```python
from build123d import *

# Parameters (mm, degrees)
SKETCH_1_W          = 175
SKETCH_1_H          = 63
EXTRUDE_1_DEPTH     = 5
CUT_EXTRUDE_1_DEPTH = 5
CHAMFER_1_SIZE      = 15
CHAMFER_2_SIZE      = 5
EXTRUDE_START       = -7
EXTRUDE_2_DEPTH     = 25
EXTRUDE_START_2     = -12
SKETCH_5_W          = 68
SKETCH_5_H          = 5
SKETCH_5_W_2        = 70
EXTRUDE_4_DEPTH     = 2
FILLET_1_R          = 3
FILLET_2_R          = 3
FILLET_3_R          = 1


with BuildPart() as part:
    # 草图1 → 凸台-拉伸1 (new body)
    with BuildSketch(Plane.XY):
        with Locations((0, 24.5)):
            Rectangle(SKETCH_1_W, SKETCH_1_H)
    extrude(amount=EXTRUDE_1_DEPTH)

    # 草图2 → 切除-拉伸1 (cut)
    with BuildSketch(Plane.XY.offset(5)):
        Polygon((-75, 56), (-4, 56), (-4, 43.171572875), (-10.171572875, 37), (-68.828427125, 37), (-75, 43.171572875), align=None)
    extrude(amount=-CUT_EXTRUDE_1_DEPTH, mode=Mode.SUBTRACT)

    # 倒角1
    chamfer_1_edges = [part.edges().sort_by_distance(p)[0] for p in [
        (87.5, -7, 2.5),
        (-87.5, -7, 2.5),
    ]]
    chamfer(chamfer_1_edges, length=CHAMFER_1_SIZE)

    # 倒角2
    chamfer_2_edges = [part.edges().sort_by_distance(p)[0] for p in [
        (-87.5, 56, 2.5),
        (87.5, 56, 2.5),
    ]]
    chamfer(chamfer_2_edges, length=CHAMFER_2_SIZE)

    # 草图4 → 凸台-拉伸2 (add)
    with BuildSketch(Plane.XZ.offset(7).offset(EXTRUDE_START)):
        Polygon((-23.5, -3), (-53.5, -3), (-51.767949192, 0), (-25.232050808, 0), align=None)
        Polygon((23.5, -3), (25.232050808, 0), (51.767949192, 0), (53.5, -3), align=None)
    extrude(amount=-EXTRUDE_2_DEPTH)

    # 草图5 → 凸台-拉伸4 (add)
    with BuildSketch(Plane(origin=(0, 37, 0), x_dir=(1, 0, 0), z_dir=(0, 1, 0)).offset(EXTRUDE_START_2)):
        with Locations((-39.5, 2.5)):
            Rectangle(SKETCH_5_W, SKETCH_5_H)
        with Locations((38.5, 2.5)):
            Rectangle(SKETCH_5_W_2, SKETCH_5_H)
    extrude(amount=-EXTRUDE_4_DEPTH)

    # 圆角1
    fillet_1_edges = [part.edges().sort_by_distance(p)[0] for p in [
        (-4, 43.171572875, 2.5),
        (-10.171572875, 37, 2.5),
        (-68.828427125, 37, 2.5),
        (-75, 43.171572875, 2.5),
        (-75, 56, 2.5),
        (-4, 56, 2.5),
        (72.5, -7, 2.5),
        (-72.5, -7, 2.5),
        (-87.5, 8, 2.5),
        (87.5, 8, 2.5),
        (82.5, 56, 2.5),
        (87.5, 51, 2.5),
        (-82.5, 56, 2.5),
    ]]
    fillet(fillet_1_edges, radius=FILLET_1_R)

    # 圆角2
    fillet_2_edges = [part.edges().sort_by_distance(p)[0] for p in [
        (-87.5, 51, 2.5),
    ]]
    fillet(fillet_2_edges, radius=FILLET_2_R)

    # 圆角3
    fillet_3_edges = [part.edges().sort_by_distance(p)[0] for p in [
        (40.128679656, 56, 5),
        (40.128679656, 56, 0),
        (87.5, 29.5, 5),
        (85, 53.5, 5),
        (-4, 48.707106781, 5),
        (-7.085786438, 40.085786438, 5),
        (-39.5, 37, 5),
        (-71.914213562, 40.085786438, 5),
        (-75, 48.707106781, 5),
        (-79.628679656, 56, 5),
        (-85, 53.5, 5),
        (-80, 0.5, 5),
        (0, -7, 5),
        (80, 0.5, 5),
        (-82.40540961, 55.771638598, 5),
        (-87.271638598, 8.09459039, 5),
        (-72.40540961, -6.771638598, 5),
        (82.40540961, 55.771638598, 5),
        (87.271638598, 50.90540961, 5),
        (87.271638598, 8.09459039, 5),
        (72.40540961, -6.771638598, 5),
        (-75.878679656, 55.121320344, 5),
        (-3.121320344, 55.121320344, 5),
        (-4, 48.707106781, 0),
        (85, 53.5, 0),
        (87.5, 29.5, 0),
        (80, 0.5, 0),
        (0, -7, 0),
        (-80, 0.5, 0),
        (-79.628679656, 56, 0),
        (-75, 48.707106781, 0),
        (-71.914213562, 40.085786438, 0),
        (-39.5, 37, 0),
        (-7.085786438, 40.085786438, 0),
        (-82.40540961, 55.771638598, 0),
        (-87.271638598, 8.09459039, 0),
        (-72.40540961, -6.771638598, 0),
        (82.40540961, 55.771638598, 0),
        (87.271638598, 50.90540961, 0),
        (87.271638598, 8.09459039, 0),
        (72.40540961, -6.771638598, 0),
        (-75.878679656, 55.121320344, 0),
        (-3.121320344, 55.121320344, 0),
        (-4.228361402, 43.266163265, 5),
        (-4.228361402, 43.266163265, 0),
        (-10.266163265, 37.228361402, 5),
        (-10.266163265, 37.228361402, 0),
        (-68.733836735, 37.228361402, 5),
        (-68.733836735, 37.228361402, 0),
        (-74.771638598, 43.266163265, 5),
        (-74.771638598, 43.266163265, 0),
        (-87.5, 29.5, 0),
        (-87.5, 29.5, 5),
        (-85, 53.5, 0),
        (-87.271638598, 50.90540961, 0),
        (-87.271638598, 50.90540961, 5),
    ]]
    fillet(fillet_3_edges, radius=FILLET_3_R)


solid = part.part
```
Input: part model. Units: mm. Frame: model coordinates. A direction names the side the tool comes from. Give positions to 0.01 mm unless a question says otherwise; leave off trailing zeros. Order: outer loops, then holes, each group sorted by start corner. A loop starts at its lowest first (then second) coordinate and runs counter-clockwise, first axis right, second up.
1. Line query: probe 1 along Y at (x, z) = (-21.5, -4.5); probe 2 along Z at (x, y) = (-49.5, 10.5); probe 3 along Z at (x, y) = (-49.5, 29). Output: solid intervals per line, ascending.
Computed:
probe 1: y = 23 to 25
probe 2: z = -3 to 5
probe 3: z = 0 to 5
2. Cut plane A-A (y = 19). Return loops of the section in (x, z), and give its area (3 significant figures).
Computed:
outline: (-87.5, 1) arc R1 ccw to (-86.5, 0) - (-51.77, 0) - (-53.5, -3) - (-23.5, -3) - (-25.23, 0) - (25.23, 0) - (23.5, -3) - (53.5, -3) - (51.77, 0) - (86.5, 0) arc R1 ccw to (87.5, 1) - (87.5, 4) arc R1 ccw to (86.5, 5) - (-86.5, 5) arc R1 ccw to (-87.5, 4) - close
area: 1,040 mm2
3. Cut plane C-C (x = 65). Return loops of the section in (y, z).
Computed:
outline: (-7, 1) arc R1 ccw to (-6, 0) - (23, 0) - (23, -5) - (25, -5) - (25, 0) - (55, 0) arc R1 ccw to (56, 1) - (56, 4) arc R1 ccw to (55, 5) - (-6, 5) arc R1 ccw to (-7, 4) - close
4. Cut plane B-B (z = -1.5). Return loops of the section in (x, y).
Computed:
outline: (-73.5, 23) - (-52.63, 23) - (-52.63, 0) - (-24.37, 0) - (-24.37, 23) - (-5.5, 23) - (-5.5, 25) - (-73.5, 25) - close; (3.5, 23) - (24.37, 23) - (24.37, 0) - (52.63, 0) - (52.63, 23) - (73.5, 23) - (73.5, 25) - (3.5, 25) - close
5. Cut plane D-D (y = 30). Return loops of the section in (x, z).
Computed:
outline: (-87.5, 1) arc R1 ccw to (-86.5, 0) - (86.5, 0) arc R1 ccw to (87.5, 1) - (87.5, 4) arc R1 ccw to (86.5, 5) - (-86.5, 5) arc R1 ccw to (-87.5, 4) - close
6. Set-up query: faces 1 (the face through (-38, 11, -3)), 2 (the face through (-71.88, 40.05, 2.52)), 3 (the face through (-87.5, 29, 2)). Return all of +Z, -Z, +X, -X, +Y, -Y with unobstructed straight access to the full face (end or side cutting, diameter ignored); none if empty.
Computed:
face 1: -Z, +X, -X, -Y
face 2: +Z, -Z, +Y
face 3: +Z, -Z, -X, +Y, -Y
7. Draft query along Z for faces 4 (the face through (24.354, 11.339, -1.521)), 5 (the face through (-80, 56, 2)), 6 (the face through (84.81, 53.265, 0.285)). Return one class per face: released by +Z, released by -Z, zero draft, split by the parting line, or undercut.
Computed:
face 4: undercut
face 5: zero draft
face 6: released by -Z
8. Pin query (flat end, axial travel): pin 1 Ø1 at (y, z) = (24, -2.5) entering from +X; pin 2 Ø11.5 at (x, y) = (-43.5, 14) entering from -Z; pin 3 Ø4 at (x, z) = (42, -3.5) entering from +Y; pin 4 Ø2.5 at (y, z) = (50.5, 2.5) entering from -X. Return the tip coordinate at first contact, or that it passes through.
Computed:
pin 1: stops at x = 73.5
pin 2: stops at z = -3
pin 3: stops at y = 25
pin 4: stops at x = -87.5
